from build123d import *

# Parameters (mm, degrees)
BOSS_EXTRU_1_DEPTH      = 11
ESQUISSE2_R             = 2.25
ENL_V_MAT_EXTRU_1_DEPTH = 13.681186853


with BuildPart() as part:
    # Esquisse1 → Boss.-Extru.1 (new body)
    with BuildSketch(Plane.XY):
        Polygon((2.500951888, 4.75), (-2.5, 4.75), (-2.75, 4.75), (-5.25, 2.25), (-4.5, 2.25), (-2.5, 2.25), (-2.5, 1.25), (2.500951888, 1.25), (2.500951888, 2.25), (4.5, 2.25), (5.25, 2.25), (2.750951888, 4.75), align=None)
    extrude(amount=BOSS_EXTRU_1_DEPTH)

    # Esquisse2 → Enlèv. mat.-Extru.1 (cut, through all)
    with BuildSketch(Plane.XZ.offset(-1.25)):
        with Locations(Location((0.000951888, 5.5, 0), (0, 0, 270))):
            Circle(ESQUISSE2_R)
    extrude(amount=-ENL_V_MAT_EXTRU_1_DEPTH, mode=Mode.SUBTRACT)


solid = part.part
Geometry check sheet. Reference: the model listing, model coordinates, mm. A direction names the side the tool comes from. Round coordinates to 2 decimals unless told otherwise and drop trailing zeros. Write each loop counter-clockwise with the first axis right and the second up, starting at its lowest first coordinate (ties: lowest second). Pieces come first, ordered by that corner, then holes. Notation, with made-up numbers: (43.5, -22) - (66.5, -22) arc R13 cw to (66.5, -17) - close; hole circle Ø5 at (-35, -11.5). An arc over 180 degrees is marked (long way). One line per item, written item: value.
1. Mould release check, pull along Z, two halves, no side actions. Record for faces 4 (the face through (0.677, 2.976, 3.354)), 5 (the face through (0, 3, 11)), 6 (the face through (0, 1.25, 8)): released by +Z, released by -Z, zero draft, split by the parting line, or undercut.
The answers:
face 4: undercut
face 5: released by +Z
face 6: zero draft
2. Scan lines: L1, parallel to Z at x = 0, y = 1.85; L2, parallel to Y at x = 4.25, z = 2.25; L3, parallel to X at y = 3, z = 5.5. Record each from-to range of solid material in increasing order.
The answers:
L1: z = 0 to 3.25, 7.75 to 11
L2: y = 2.25 to 3.25
L3: x = -4.5 to -2.25, 2.25 to 4.5
3. Cross-section at C-C on x = 1.75. Record the boundary of the cut face in (y, z).
The answers:
outline: (1.25, 0) - (4.75, 0) - (4.75, 4.08) - (1.25, 4.08) - close; (1.25, 6.92) - (4.75, 6.92) - (4.75, 11) - (1.25, 11) - close
4. Depth check by flat-ended pin: pin 1 Ø2 at (x, z) = (-3, 9.5) entering from +Y; pin 2 Ø2 at (x, z) = (-4, 7) entering from -Y; pin 3 Ø2 at (y, z) = (4.5, 5.5) entering from -X; pin 4 Ø1.1 at (y, z) = (1.5, 7) entering from -X. Enter the tip coordinate at first touch or a pass-through.
The answers:
pin 1: stops at y = 4.75
pin 2: stops at y = 2.25
pin 3: stops at x = -4
pin 4: stops at x = -2.5
5. Cross-section at D-D on y = 1.85. Record the boundary of the cut face in (x, z), and give its area (3 significant figures).
The answers:
outline: (-2.5, 0) - (2.5, 0) - (2.5, 11) - (-2.5, 11) - close; hole circle Ø4.5 at (0, 5.5)
area: 39.1 mm^2
6. Set-up check for faces 1 (the face through (4, 2.25, 5)), 2 (the face through (0, 3, 0)), 3 (the face through (-2.5, 2, 5)): record each of +Z, -Z, +X, -X, +Y, -Y from which the full face is reachable in a straight line by a thin tool's end or side.
The answers:
face 1: +Z, -Z, +X, -Y
face 2: -Z, +X, -X, +Y, -Y
face 3: +Z, -Z, -X, -Y
7. Cross-section at A-A on z = 5.5. Record the boundary of the cut face in (x, y).
The answers:
outline: (-5.25, 2.25) - (-2.5, 2.25) - (-2.5, 1.25) - (-2.25, 1.25) - (-2.25, 4.75) - (-2.75, 4.75) - close; (2.25, 1.25) - (2.5, 1.25) - (2.5, 2.25) - (5.25, 2.25) - (2.75, 4.75) - (2.25, 4.75) - close
8. Cross-section at B-B on z = 2.5. Record the boundary of the cut face in (x, y), and give its area (3 significant figures).
The answers:
outline: (-5.25, 2.25) - (-2.5, 2.25) - (-2.5, 1.25) - (2.5, 1.25) - (2.5, 2.25) - (5.25, 2.25) - (2.75, 4.75) - (-2.75, 4.75) - close
area: 25.0 mm^2
